```python
from build123d import *

# Parameters (mm, degrees)
F5_DEPTH  = 2.54
F7_DEPTH  = 2.54
F9_DEPTH  = 2.54
F11_DEPTH = 2.54
F14_R     = 1.27
F15_DEPTH = 30.0736
F16_R     = 42.413221
F16_R_2   = 20.955
F17_DEPTH = 25.4


with BuildPart() as f5:
    # F4 (on offset) → F5 (new body)
    with BuildSketch(Plane.YZ.offset(20.32)):
        Polygon((7.62, 0), (0, 0), (-0.671806, -3.81), align=None)
    extrude(amount=-F5_DEPTH)



with BuildPart() as f7:
    # F6 (on offset) → F7 (new body)
    with BuildSketch(Plane.YZ.offset(-20.32)):
        Polygon((0.671806, -3.81), (0, 0), (-7.62, 0), align=None)
    extrude(amount=F7_DEPTH)


with BuildPart() as f9:
    # F8 (on offset) → F9 (new body)
    with BuildSketch(Plane.XZ.offset(-20.32)):
        Polygon((0.671806, -3.81), (0, 0), (-7.62, 0), align=None)
    extrude(amount=F9_DEPTH)


with BuildPart() as f11:
    # F10 (on offset) → F11 (new body)
    with BuildSketch(Plane.XZ.offset(20.32)):
        Polygon((7.62, 0), (0, 0), (-0.671806, -3.81), align=None)
    extrude(amount=-F11_DEPTH)


with BuildPart() as f5_1:
    add(f5.part)

    add(f7.part)  # F13 merges F7

    add(f9.part)  # F13 merges F9

    add(f11.part)  # F13 merges F11
    # F12 (on Front) → F13 (revolve)
    with BuildSketch(Plane.XZ):
        Polygon((-21.59, 0), (-16.51, 0), (0, 2.911158), (0, 40.299149), (-10.16, 40.299149), (-10.16, 33.949149), (-5.08, 33.949149), (-5.08, 8.549149), (-21.59, 2.54), align=None)
    revolve(axis=Axis((0, 0, 23.632418), (0, 0, 1)))

    # F14 (on offset) → F15 (cut)
    with BuildSketch(Plane.XZ.offset(20.32)):
        with Locations((0, 21.249149)):
            Circle(F14_R)
    extrude(amount=-F15_DEPTH, mode=Mode.SUBTRACT)

    # F16 (on Top) → F17 (cut)
    with BuildSketch(Plane.XY):
        Circle(F16_R)
        Circle(F16_R_2, mode=Mode.SUBTRACT)
    extrude(amount=-F17_DEPTH, mode=Mode.SUBTRACT)


solid = f5_1.part
```
Source: CAD feature listing. Evaluate the final solid. Frame: model axes, mm. A direction names the side the tool comes from. Give positions to 0.01 mm unless a question says otherwise; leave off trailing zeros. Loops run counter-clockwise (first coordinate to the right, second up) from the corner with the lowest first, then second, coordinate; pieces in that order, holes last. Notation, with made-up numbers: M 73,31 L 115,31 A5 ccw 115,38 Z; hole C 47,79.25 d7. An arc over 180 degrees is marked long. Put each result on its own line as item: value.
Q1. Reachability of faces 5 (the cylindrical face through (-4.845, -1.526, 21.071)), 6 (the cylindrical face through (6.09, -20.05, -0.44)), 7 (the flat face through (20.32, 2, -1)), 8 (the cylindrical face through (1.323, -10.074, 37.08)) from +Z, -Z, +X, -X, +Y, -Y: full face, straight path, thin tool, end or side. Return the list, or none.
Response values:
face 5: none
face 6: -Z, +X, -Y
face 7: -Z, +X, +Y, -Y
face 8: +Z
Q2. Mould query, pull axis Z, two halves, no side actions, for faces 1 (the flat face through (-19.07, -3.53, -1.88)), 2 (the conical face through (6.11, -0.27, 8.17)), 3 (the flat face through (-2, 20.32, -1)), 4 (the flat face through (5, 2, 33.949)). Classes: released by +Z, released by -Z, zero draft, split by the parting line, or undercut.
Response values:
face 1: released by -Z
face 2: undercut
face 3: zero draft
face 4: undercut
Q3. Line query: probe 1 along Z at (x, y) = (0, 0); probe 2 along Z at (x, y) = (0, -2); probe 3 along Y at (x, z) = (0.5, 31). Output: solid intervals per line, ascending. Write a range as [from, to].
Response values:
probe 1: z = [2.91, 19.98], [22.52, 40.3]
probe 2: z = [2.56, 19.98], [22.52, 40.3]
probe 3: y = [-5.06, 5.06]
Q4. Section B-B (z = 35.5). Return the cut outline in (x, y).
Response values:
outline: C 0,0 d20.32
Q5. Pin query (flat end, axial travel): P1, Ø10, axis at y = 7.5, z = 23.5, coming from the +X side; P2, Ø1.1, axis at y = 2.5, z = -1.5, coming from the +X side; P3, Ø3, axis at x = 12.5, y = -16.5, coming from the +Z side; P4, Ø10, axis at y = 13.5, z = 12.5, coming from the -X side (1 decimal). Return the tip coordinate at first contact, or that it passes through.
Response values:
P1: stops at x = 4.42
P2: stops at x = 20.32
P3: stops at z = 3.41
P4: passes through
Q6. Section A-A (z = 14.5). Return the cut outline in (x, y).
Response values:
outline: C 0,0 d10.16
